Source: three-view drawing plus pictorial views. Frame: mm from the lowest corner of the part. A direction names the side the tool comes from. Give positions to 0.01 mm unless a question says otherwise; leave off trailing zeros. Loops run counter-clockwise (first coordinate to the right, second up) from the corner with the lowest first, then second, coordinate; pieces in that order, holes last.
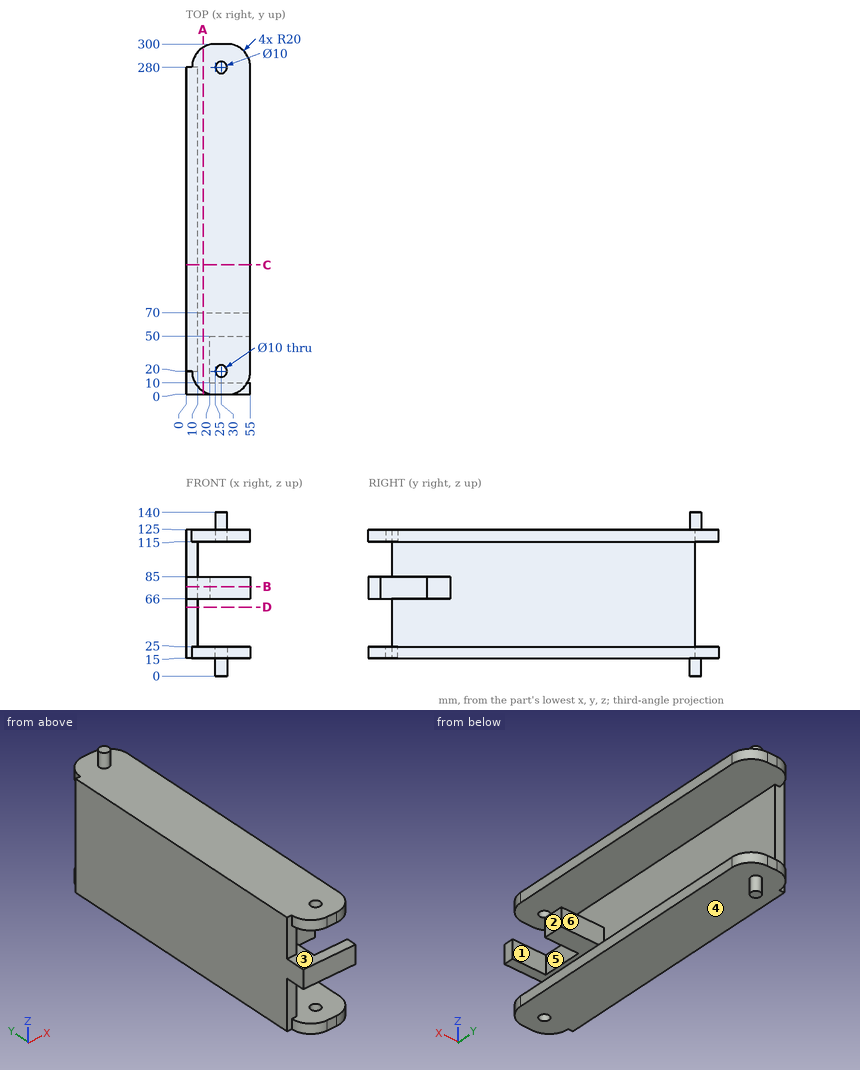
1) Pull-direction query (Y, two-part tool) for the marked faces 4, 5 and 6; classes: released by +Y, released by -Y, zero draft, split by the parting line, or undercut.
Checks:
face 4: zero draft
face 5: undercut
face 6: released by +Y
2) Reachability of the marked faces 1, 2 and 3 from +Z, -Z, +X, -X, +Y, -Y: full face, straight path, thin tool, end or side. Return the list, or none.
Checks:
face 1: +X
face 2: +Z, -Z, +X, +Y, -Y
face 3: +X, -Y
3) Cut plane B-B (z = 76.5). Return loops of the section in (x, y), and give its area (3 significant figures).
Checks:
outline: (0, 0) - (55, 0) - (55, 10) - (20, 10) - (20, 50) - (55, 50) - (55, 70) - (10, 70) - (10, 280) - (0, 280) - close
area: 4,550 mm2
4) Ray query, probe 1 along Z at (x, y) = (16, 63.5); probe 2 along Y at (x, z) = (30, 120.5); probe 3 along Z at (x, y) = (38.5, 147). Return the intervals inside material, ascending.
Checks:
probe 1: z = 15 to 25, 66 to 85, 115 to 125
probe 2: y = 0 to 15, 25 to 300
probe 3: z = 15 to 25, 115 to 125
5) Cut plane C-C (y = 111). Return loops of the section in (x, z).
Checks:
outline: (0, 15) - (55, 15) - (55, 25) - (10, 25) - (10, 115) - (55, 115) - (55, 125) - (0, 125) - close
6) Cut plane D-D (z = 59). Return loops of the section in (x, y).
Checks:
outline: (0, 20) - (10, 20) - (10, 280) - (0, 280) - close
7) Cut plane A-A (x = 14.5). Return loops of the section in (y, z), and give its area (3 significant figures).
Checks:
outline: (0, 66) - (70, 66) - (70, 85) - (0, 85) - close; (2.98, 15) - (297.02, 15) - (297.02, 25) - (2.98, 25) - close; (2.98, 115) - (297.02, 115) - (297.02, 125) - (2.98, 125) - close
area: 7,210 mm2
8) Contact query for flat-ended pins moving along their axis: P1, Ø8, axis at y = 82, z = 36, coming from the +X side; P2, Ø10, axis at x = 26, y = 57, coming from the +Z side; P3, Ø9.5, axis at y = 32, z = 78, coming from the +X side. Output: stop coordinate, or through.
Checks:
P1: stops at x = 10
P2: stops at z = 125
P3: stops at x = 20
